Autodesk Inventor part; units mm, degrees
ref_plane "YZ Plane" through (0, 0, 0) normal (1, 0, 0) x (0, 1, 0)
ref_plane "XZ Plane" through (0, 0, 0) normal (0, 1, 0) x (-1, 0, 0)
ref_plane "XY Plane" through (0, 0, 0) normal (0, 0, 1) x (1, 0, 0)
sketch "Sketch1: base" plane through (0, 0, 0) normal (0, 0, 1) x (1, 0, 0)
  line L0 (-22.5, 22.5) -> (22.5, 22.5)
  line L1 (22.5, 22.5) -> (22.5, -22.5)
  line L2 (22.5, -22.5) -> (-22.5, -22.5)
  line L3 (-22.5, -22.5) -> (-22.5, 22.5)
  circle A0 centre (0, 0) radius 14.875
  line L4 (-16, 16) -> (16, 16) construction
  line L5 (16, 16) -> (16, -16) construction
  line L6 (16, -16) -> (-16, -16) construction
  line L7 (-16, -16) -> (-16, 16) construction
  circle A1 centre (16, 16) radius 1.8 construction
  circle A2 centre (16, 16) radius 3.25 construction
  point P0 (22.5, 0)
  point P1 (0, 22.5)
  point P2 (0, 16)
  point P3 (-16, 0)
  dimension "d0" = 29.75
  dimension "d1" = 45
  dimension "d4" = 32
  dimension "d19" = 6.5
  dimension "d20" = 3.6
  dimension "d21" = 6.5
extrude "Ex1: base" add sketch "Sketch1: base" along normal blind 4
hole "Hole1: M3 screws" at (-16, 16, 0) at (16, 16, 0) at (-16, -16, 0) at (16, -16, 0) direction (0, 0, 1) diameter 3.7 end through all counterbore diameter 6.5 counterbore depth 3
fillet "Fillet1" radius 2 8 edges at (0, 22.5, 0) (22.5, 0, 0) (22.5, 22.5, 2) (-22.5, 0, 0) (0, -22.5, 0) (22.5, -22.5, 2) (-22.5, -22.5, 2) (-22.5, 22.5, 2)
sketch "Sketch2: text" plane through (0, 0, 0) normal (0, 0, -1) x (-1, 0, 0)
  line L0 (-9.5, 19) -> (-6, 19) construction
  line L1 (-6, 19) -> (-6, 15.5) construction
  line L2 (-6, 15.5) -> (-9.5, 15.5) construction
  line L3 (-9.5, 15.5) -> (-9.5, 19) construction
  line L4 (22.5, 22.5) -> (-22.5, 22.5) construction
  line L5 (-22.5, 22.5) -> (-22.5, -22.5) construction
  line L6 (22.5, -22.5) -> (22.5, 22.5) construction
  line L7 (-22.5, -22.5) -> (22.5, -22.5) construction
  circle A0 centre (-16, 16) radius 3.25 construction
  circle A1 centre (-16, 16) radius 1.8 construction
  line L8 (16, 16) -> (-16, 16) construction
  circle A2 centre (0, 0) radius 14.875 construction
  circle A3 centre (0, 0) radius 14.875 construction
  line L9 (-12.2062, 18.3737) -> (-10.7625, 18.3737)
  line L10 (-10.7625, 18.3737) -> (-10.0551, 16.0782)
  line L11 (-10.0551, 16.0782) -> (-9.3284, 18.3737)
  line L12 (-9.3284, 18.3737) -> (-7.9281, 18.3737)
  line L13 (-7.9281, 18.3737) -> (-9.468, 14.75)
  line L14 (-9.468, 14.75) -> (-10.7, 14.75)
  line L15 (-10.7, 14.75) -> (-12.2062, 18.3737)
  line L16 (-6.3111, 18.3063) -> (-7.6249, 18.5421)
  spline S0 degree 2 poles (-7.6249, 18.5421) (-7.4613, 19.1677) (-6.5325, 19.8366) (-5.6807, 19.8366) knots 0 0 0 1 2 2 2
  spline S1 degree 2 poles (-5.6807, 19.8366) (-4.699, 19.8366) (-3.828, 19.1051) (-3.828, 18.5565) knots 0 0 0 1 2 2 2
  spline S2 degree 2 poles (-3.828, 18.5565) (-3.828, 18.2293) (-4.1841, 17.7048) (-4.545, 17.5075) knots 0 0 0 1 2 2 2
  spline S3 degree 2 poles (-4.545, 17.5075) (-4.2514, 17.4353) (-4.0974, 17.339) knots 0 0 0 1 1 1
  spline S4 degree 2 poles (-4.0974, 17.339) (-3.8472, 17.185) (-3.5729, 16.6846) (-3.5729, 16.3381) knots 0 0 0 1 2 2 2
  spline S5 degree 2 poles (-3.5729, 16.3381) (-3.5729, 15.9001) (-4.0301, 15.0965) (-4.8867, 14.6634) (-5.5893, 14.6634) knots 0 0 0 1 2 3 3 3
  spline S6 degree 2 poles (-5.5893, 14.6634) (-6.2678, 14.6634) (-7.057, 14.9858) (-7.5671, 15.6018) (-7.7019, 16.0686) knots 0 0 0 1 2 3 3 3
  line L17 (-7.7019, 16.0686) -> (-6.3111, 16.2514)
  spline S7 degree 2 poles (-6.3111, 16.2514) (-6.2293, 15.8328) (-5.8876, 15.5103) (-5.623, 15.5103) knots 0 0 0 1 2 2 2
  spline S8 degree 2 poles (-5.623, 15.5103) (-5.3438, 15.5103) (-4.9733, 15.9194) (-4.9733, 16.2611) knots 0 0 0 1 2 2 2
  spline S9 degree 2 poles (-4.9733, 16.2611) (-4.9733, 16.6124) (-5.3294, 16.9925) (-5.6374, 16.9925) knots 0 0 0 1 2 2 2
  spline S10 degree 2 poles (-5.6374, 16.9925) (-5.801, 16.9925) (-6.0849, 16.9107) knots 0 0 0 1 1 1
  line L18 (-6.0849, 16.9107) -> (-6.0128, 17.9069)
  spline S11 degree 2 poles (-6.0128, 17.9069) (-5.8973, 17.8876) (-5.8347, 17.8876) knots 0 0 0 1 1 1
  spline S12 degree 2 poles (-5.8347, 17.8876) (-5.5604, 17.8876) (-5.1947, 18.2341) (-5.1947, 18.4747) knots 0 0 0 1 2 2 2
  spline S13 degree 2 poles (-5.1947, 18.4747) (-5.1947, 18.7009) (-5.469, 18.9752) (-5.7048, 18.9752) knots 0 0 0 1 2 2 2
  spline S14 degree 2 poles (-5.7048, 18.9752) (-5.9502, 18.9752) (-6.2582, 18.6769) (-6.3111, 18.3063) knots 0 0 0 1 2 2 2
  point P0 (-7.75, 19)
  point P1 (0, 22.5)
  dimension "d23" = 3.5
  dimension "d24" = 3.5
  dimension "d29" = 13
extrude "Ex3: text" cut sketch "Sketch2: text" against normal blind 1
properties part number "cage_inside_03"
Geometry check sheet. Reference: the model listing, model coordinates, mm. A direction names the side the tool comes from. Coordinates: 2 decimals unless noted, no trailing zeros. Order: outer loops, then holes, each group sorted by start corner. A loop starts at its lowest first (then second) coordinate and runs counter-clockwise, first axis right, second up. Notation, with made-up numbers: (43, -26) - (85, -26) arc R18 cw to (85, -19) - close; hole circle Ø8 at (-11, 34.25). An arc over 180 degrees is marked (long way). Answer as a JSON object with one key per item and string values. Group by question number.
Item 1: Sectioned sample at A-A, the plane y = -16. Record the cut outline in (x, z), and give its area (3 significant figures).
Item 2: Sectioned sample at D-D, the plane x = 13.5. Record the cut outline in (y, z).
Item 3: Scan lines: probe 1 along X at (y, z) = (16, 3.35); probe 2 along Y at (x, z) = (16, 1.8); probe 3 along X at (y, z) = (16, 2.05). Record each from-to range of solid material in increasing order.
Item 4: Depth check by flat-ended pin: pin 1 Ø2 at (x, y) = (-17.5, -16) entering from -Z. Enter the tip coordinate at first touch or a pass-through.
Item 5: Sectioned sample at C-C, the plane y = 0. Record the cut outline in (x, z) (3 decimals).
Item 6: Tool access check on faces 5 (the face through (9, -13, 0)), 6 (the face through (18.1, 16, 3)). Record the directions out of +Z, -Z, +X, -X, +Y, -Y that give a thin tool (end or side, any length) a straight path to the whole face; none if there is none.
Item 7: Draft check along Y on faces 1 (the face through (18.1, -16, 3)), 2 (the face through (10.1, 14.75, 0.5)), 3 (the face through (-21.9, 0.29, 0.57)), 4 (the face through (0.29, 21.9, 0.57)). Enter one of: +Y half, -Y half, draft (parallel to the pull), parting line (faces both ways), or undercut.
Resolved:
{
 "1": {"outline": "(-22.5, 2) arc R2 ccw to (-20.5, 0) - (-19.25, 0) - (-19.25, 3) - (-17.85, 3) - (-17.85, 4) - (-22.5, 4) - close; (-14.15, 3) - (-12.75, 3) - (-12.75, 0) - (12.75, 0) - (12.75, 3) - (14.15, 3) - (14.15, 4) - (-14.15, 4) - close; (17.85, 3) - (19.25, 3) - (19.25, 0) - (20.5, 0) arc R2 ccw to (22.5, 2) - (22.5, 4) - (17.85, 4) - close", "area": "132 mm^2"},
 "2": {"outline": "(-22.5, 2) arc R2 ccw to (-20.5, 0) - (-18.08, 0) - (-18.08, 3) - (-13.92, 3) - (-13.92, 0) - (-6.25, 0) - (-6.25, 4) - (-22.5, 4) - close; (6.25, 0) - (13.92, 0) - (13.92, 3) - (18.08, 3) - (18.08, 0) - (20.5, 0) arc R2 ccw to (22.5, 2) - (22.5, 4) - (6.25, 4) - close"},
 "3": {"probe 1": "-22.5 to -17.85, -14.15 to 14.15, 17.85 to 22.5", "probe 2": "-22.49 to -19.25, -12.75 to 12.75, 19.25 to 22.49", "probe 3": "-22.5 to -19.25, -12.75 to 12.75, 19.25 to 22.5"},
 "4": {"pin 1": "z = 3"},
 "5": {"outline": "(-22.5, 2) arc R2 ccw to (-20.5, 0) - (-14.875, 0) - (-14.875, 4) - (-22.5, 4) - close; (14.875, 0) - (20.5, 0) arc R2 ccw to (22.5, 2) - (22.5, 4) - (14.875, 4) - close"},
 "6": {"face 5": "-Z, +X, -X, +Y, -Y", "face 6": "-Z"},
 "7": {"face 1": "undercut", "face 2": "undercut", "face 3": "draft", "face 4": "+Y half"}
}
